Input: part model. Units: mm. Frame: model coordinates. A direction names the side the tool comes from. Coordinates: 2 decimals unless noted, no trailing zeros. Write each loop counter-clockwise with the first axis right and the second up, starting at its lowest first coordinate (ties: lowest second). Pieces come first, ordered by that corner, then holes. Notation, with made-up numbers: (70.25, 81) - (108.25, 81) arc R16 ccw to (108.25, 87) - close; hole circle Ø7 at (59.25, 35.25). An arc over 180 degrees is marked (long way). Use a Markdown table: item, result. Add a question column.
Q1. Material intervals for probe 1 along Z at (x, y) = (-24, -12); probe 2 along Z at (x, y) = (-10, -23.25); probe 3 along Z at (x, y) = (24.5, -12.5), sorted ascending. Write a range as from..to.
Q2. Section query C-C (y = -8). Return the cut outline in (x, z).
Q3. Pin query (flat end, axial travel): P1, Ø1.5, axis at x = 1, z = 11, coming from the -Y side; P2, Ø5, axis at x = -24, z = 15, coming from the +Y side; P3, Ø2.5, axis at x = -24, z = 5, coming from the -Y side; P4, Ø4.5, axis at x = 24, z = 15, coming from the -Y side. Return the tip coordinate at first contact, or that it passes through.
Q4. Section query D-D (x = 2). Return the cut outline in (y, z).
Q5. Section query B-B (x = 17). Return the cut outline in (y, z).
Q6. Section query A-A (x = 24). Return the cut outline in (y, z).
Q7. Mould query, pull axis X, two halves, no side actions, for faces 1 (the face through (-22, -12, 15)), 2 (the face through (14, -20, 10)), 3 (the face through (-18, -18.42, 2)). Classes: released by +X, released by -X, zero draft, split by the parting line, or undercut.
Q8. Set-up query: faces 4 (the face through (-5, -22.7, 8.4)), 5 (the face through (-20, 3, 10)), 6 (the face through (-18, -18.42, 18)). Return all of +Z, -Z, +X, -X, +Y, -Y with unobstructed straight access to the full face (end or side cutting, diameter ignored); none if empty.
Autodesk Inventor part; units mm, degrees
ref_plane "РабПлоскость1" through (0, 0, 10) normal (0, 0, 1) x (1, 0, 0)
ref_plane "РабПлоскость3" through (0, -10.9196, 0) normal (1, 0, 0) x (0, 0, -1)
ref_plane "YZ Plane" through (0, 0, 0) normal (1, 0, 0) x (0, 1, 0)
sketch "Эскиз1" plane through (0, 0, 0) normal (0, 0, 1) x (1, 0, 0)
  line L0 (0, 17.0804) -> (20, 17.0804)
  line L1 (0, 24.5911) -> (0, -44.9718)
  line L2 (14, -21.4196) -> (0, -21.4196)
  line L3 (20, 17.0804) -> (20, -10.9196)
  line L4 (20, -10.9196) -> (26.75, -10.9196)
  line L5 (26.75, -10.9196) -> (26.75, -12.9196)
  line L6 (26.75, -12.9196) -> (20, -12.9196)
  line L7 (20, -12.9196) -> (20, -18.4196)
  line L8 (14, -21.4196) -> (14, -18.4196)
  line L9 (14, -18.4196) -> (20, -18.4196)
  line L10 (0, 17.0804) -> (-20, 17.0804)
  line L11 (-14, -21.4196) -> (0, -21.4196)
  line L12 (-20, 17.0804) -> (-20, -10.9196)
  line L13 (-20, -10.9196) -> (-26.75, -10.9196)
  line L14 (-26.75, -10.9196) -> (-26.75, -12.9196)
  line L15 (-26.75, -12.9196) -> (-20, -12.9196)
  line L16 (-20, -12.9196) -> (-20, -18.4196)
  line L17 (-14, -21.4196) -> (-20, -21.4196)
  line L18 (-20, -21.4196) -> (-20, -18.4196)
  point P0 (0, 0)
  dimension "d14" = 28
  dimension "d15" = 6.75
  dimension "d16" = 2
  dimension "d17" = 6
  dimension "d18" = 3
  dimension "d20" = 20
extrude "Выдавливание1" add sketch "Эскиз1" along normal blind 20
sketch "Эскиз2" plane through (20, -10.9196, 0) normal (0, 1, 0) x (1, 0, 0)
  line L0 (0, 0) -> (0, -20)
  line L1 (0, -10) -> (9.888, -10)
  arc A0 (5.7321, -4) -> (5.7321, -6) centre (4, -5) ccw
  line L2 (6.75, 0) -> (6.75, -20)
  line L3 (6, -4) -> (6.75, -4)
  line L4 (6, -6) -> (6.75, -6)
  line L5 (6, -4) -> (5.7321, -4)
  line L6 (6, -6) -> (5.7321, -6)
  point P0 (-20, 0)
  dimension "d23" = 4
  dimension "d24" = 3
  dimension "d25" = 2
extrude "Выдавливание2" cut sketch "Эскиз2" against normal through all
ref_plane "РабПлоскость1" through (0, 0, 10) normal (0, 0, 1) x (1, 0, 0)
mirror "Зеркальное отражение2" about plane through (0, 0, 10) normal (0, 0, 1) of "Выдавливание2"
ref_plane "РабПлоскость3" through (0, -10.9196, 0) normal (1, 0, 0) x (0, 0, -1)
mirror "Зеркальное отражение3" about plane through (0, -10.9196, 0) normal (1, 0, 0) of "Выдавливание2", "Зеркальное отражение2"
chamfer "Фаска1" distance 1 angle 45 4 edges at (0, 17.0804, 20) (20, 17.0804, 10) (0, 17.0804, 0) (-20, 17.0804, 10)
sketch "Эскиз3" plane through (-14, -21.4196, 0) normal (0, -1, 0) x (1, 0, 0)
  line L0 (28, 0) -> (28, 20)
  line L1 (-6, 0) -> (-6, 20)
  line L2 (-6, 20) -> (34, 20)
  circle A0 centre (4, 10) radius 10
  circle A1 centre (4, 10) radius 2.75
  circle A2 centre (4, 10) radius 5.25
  circle A3 centre (4, 10) radius 6.5
  line L3 (-6, 0) -> (-12.75, 0)
  line L4 (-6, 0) -> (4, 0)
  line L5 (-6, 20) -> (4, 20)
  line L6 (-6, 20) -> (28, 20)
  line L7 (-6, 0) -> (-6, 20)
  line L8 (-6, 0) -> (-6, 20)
  point P0 (14, 0)
  point P1 (-6, 10)
  dimension "d39" = 5.5
  dimension "d41" = 10.5
  dimension "d42" = 13
extrude "Выдавливание3" cut sketch "Эскиз3" against normal up to surface (3 mm away) contours L1 A0 L4 | L1 L2 A0
sketch "Эскиз5" plane through (14, -21.4196, 0) normal (0, -1, 0) x (1, 0, 0)
  point P0 (-14, 0)
extrude "Выдавливание4" add sketch "Эскиз3" along normal blind 1 contours A3
extrude "Выдавливание5" add sketch "Эскиз3" along normal blind 1.5 contours A2
extrude "Выдавливание6" add sketch "Эскиз3" along normal blind 6 contours A1
sketch "Эскиз6" plane through (-10, -27.4196, 10) normal (0, -1, 0) x (1, 0, 0)
  circle A0 centre (0, 0) radius 1
  point P0 (10, -10)
  dimension "d52" = 2
extrude "Выдавливание7" cut sketch "Эскиз6" against normal up to surface (9 mm away)
properties part number "Сервопривод"
Values follow:
| question | item | result |
|---|---|---|
| 1 | probe 1 | 0..3, 7..13, 17..20 |
| 1 | probe 2 | 7.25..9, 11..12.75 |
| 1 | probe 3 | 0..3.06, 6.94..13.06, 16.94..20 |
| 2 | outline | (-20, 0) - (20, 0) - (20, 20) - (-20, 20) - close |
| 3 | P1 | y = -21.42 |
| 3 | P2 | y = -10.92 |
| 3 | P3 | through |
| 3 | P4 | y = -12.92 |
| 4 | outline | (-21.42, 0) - (16.08, 0) - (17.08, 1) - (17.08, 19) - (16.08, 20) - (-21.42, 20) - close |
| 5 | outline | (-18.42, 0) - (16.08, 0) - (17.08, 1) - (17.08, 19) - (16.08, 20) - (-18.42, 20) - close |
| 6 | outline | (-12.92, 0) - (-10.92, 0) - (-10.92, 3) - (-12.92, 3) - close; (-12.92, 7) - (-10.92, 7) - (-10.92, 13) - (-12.92, 13) - close; (-12.92, 17) - (-10.92, 17) - (-10.92, 20) - (-12.92, 20) - close |
| 7 | face 1 | undercut |
| 7 | face 2 | released by +X |
| 7 | face 3 | zero draft |
| 8 | face 4 | -Y |
| 8 | face 5 | +Z, -Z, -X, +Y |
| 8 | face 6 | +Z, -X, -Y |
